from build123d import *


with BuildPart() as part:
    # Esquisse1 → Révolution1 (revolve)
    with BuildSketch(Plane.XY):
        with BuildLine():
            Line((0, 30.65), (0, 27))
            Line((0, 27), (1, 26))
            Line((1, 26), (2, 26))
            Line((2, 26), (2, 23.6))
            Line((2, 23.6), (5, 23.6))
            Line((5, 23.6), (5, 26.422161222))
            Line((5, 26.422161222), (3.149522108, 29.072161222))
            ThreePointArc((3.149522108, 29.072161222), (3.106544314, 29.570228141), (3.516339637, 29.856559314))
            Line((3.516339637, 29.856559314), (5.173152545, 30))
            Line((5.173152545, 30), (22.325638556, 30))
            Line((22.325638556, 30), (23.987869468, 29.85529344))
            ThreePointArc((23.987869468, 29.85529344), (24.395805636, 29.568829063), (24.353440423, 29.072161222))
            Line((24.353440423, 29.072161222), (22.5, 26.422161222))
            Line((22.5, 26.422161222), (22.5, 23.6))
            Line((22.5, 23.6), (25.5, 23.6))
            Line((25.5, 23.6), (25.5, 26))
            Line((25.5, 26), (26.5, 26))
            Line((26.5, 26), (27.5, 27))
            Line((27.5, 27), (27.5, 30.65))
            ThreePointArc((27.5, 30.65), (27.238547604, 31.328009544), (26.587105785, 31.65))
            Line((26.587105785, 31.65), (22.499950042, 32))
            Line((22.499950042, 32), (5, 32))
            Line((5, 32), (0.91370073, 31.64622344))
            ThreePointArc((0.91370073, 31.64622344), (0.263015483, 31.325890185), (0, 30.65))
        make_face()
    revolve(axis=Axis((0, 0, 0), (1, 0, 0)))


solid = part.part
Source: CAD feature listing. Evaluate the final solid. Frame: model axes, mm. A direction names the side the tool comes from. Round coordinates to 2 decimals unless told otherwise and drop trailing zeros. Loops run counter-clockwise (first coordinate to the right, second up) from the corner with the lowest first, then second, coordinate; pieces in that order, holes last.
Q1. Section A-A, the plane x = 15.75. Return loops of the section in (y, z).
Q2. First-contact query: P1, Ø5, axis at x = 6.5, y = 23.5, coming from the +Z side; P2, Ø3, axis at x = 21.5, y = -14, coming from the -Z side; P3, Ø3, axis at x = 11.5, y = -17, coming from the +Z side; P4, Ø16, axis at y = 0, z = -11.5, coming from the -X side. Flat tips, straight axial feed; report the tip coordinate or a pass-through.
Q3. Ray query, line 1 (Z direction, x = 10, y = 0); line 2 (X direction, y = 7, z = 24); line 3 (X direction, y = -26, z = 13). Return the intervals inside material, ascending.
Q4. Mould query, pull axis Z, two halves, no side actions, for faces 4 (the face through (0, 2.1, -27.1)), 5 (the face through (24.021, -23.577, 1.038)), 6 (the face through (13.63, -6.94, -31.24)). Classes: pulls with the +Z half, pulls with the -Z half, needs draft (parallel to the pull), parting line crosses it, or undercut.
Q5. Access query for faces 1 (the face through (1.507, -20.633, -15.821)), 2 (the face through (22.5, -10, 22)), 3 (the face through (26.007, -20.633, -15.821)). Directions: +Z, -Z, +X, -X, +Y, -Y. A direction counts if a zero-diameter tool reaches every point of the face in a straight line with its end or side. Return the directions, or none.
Solutions:
1. outline: circle Ø64 at (0, 0); hole circle Ø60 at (0, 0)
2. P1: stops at z = 24.15
2. P2: stops at z = -29.46
2. P3: stops at z = 28
2. P4: passes through
3. line 1: z = -32 to -30, 30 to 32
3. line 2: x = 2 to 5, 22.5 to 25.5
3. line 3: x = 0 to 3.15, 24.35 to 27.5
4. face 4: needs draft
4. face 5: undercut
4. face 6: parting line crosses it
5. face 1: -X
5. face 2: none
5. face 3: +X
